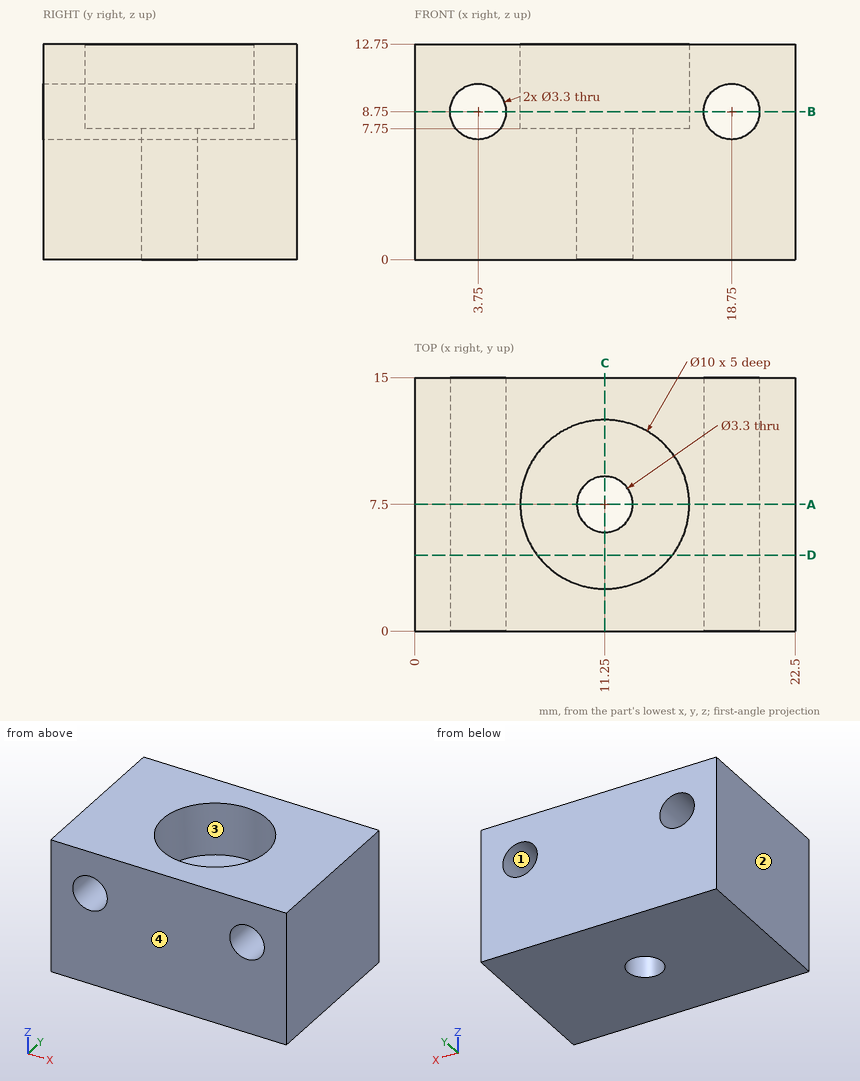
Geometry check sheet. Reference: drawing and pictorial views, mm from the part's lowest x, y, z. Coordinates: 2 decimals unless noted, no trailing zeros. Order: outer loops, then holes, each group sorted by start corner. A loop starts at its lowest first (then second) coordinate and runs counter-clockwise, first axis right, second up.
Item 1: Mould release check, pull along X, two halves, no side actions. Record for the marked faces 1, 2, 3 and 4: released by +X, released by -X, zero draft, split by the parting line, or undercut.
Item 2: Section check A-A (y = 7.5). Enter the section's corners in (x, z).
Item 3: Section check D-D (y = 4.5). Enter the section's corners in (x, z).
Item 4: Scan lines: line 1 along X through (y, z) = (10.75, 8.75); line 2 along Y through (x, z) = (11.25, 10); line 3 along X through (y, z) = (7, 8.75). Record each from-to range of solid material in increasing order.
Item 5: Section check B-B (z = 8.75). Enter the section's corners in (x, y), plus the area to 3 significant figures.
Item 6: Section check C-C (x = 11.25). Enter the section's corners in (y, z).
Check sheet entries:
1. face 1: undercut
1. face 2: released by -X
1. face 3: undercut
1. face 4: zero draft
2. outline: (0, 0) - (9.6, 0) - (9.6, 7.75) - (6.25, 7.75) - (6.25, 12.75) - (0, 12.75) - close; (12.9, 0) - (22.5, 0) - (22.5, 12.75) - (16.25, 12.75) - (16.25, 7.75) - (12.9, 7.75) - close; hole circle Ø3.3 at (3.75, 8.75); hole circle Ø3.3 at (18.75, 8.75)
3. outline: (0, 0) - (22.5, 0) - (22.5, 12.75) - (15.25, 12.75) - (15.25, 7.75) - (7.25, 7.75) - (7.25, 12.75) - (0, 12.75) - close; hole circle Ø3.3 at (3.75, 8.75); hole circle Ø3.3 at (18.75, 8.75)
4. line 1: x = 0 to 2.1, 5.4 to 7.45, 15.05 to 17.1, 20.4 to 22.5
4. line 2: y = 0 to 2.5, 12.5 to 15
4. line 3: x = 0 to 2.1, 5.4 to 6.28, 16.22 to 17.1, 20.4 to 22.5
5. outline: (0, 0) - (2.1, 0) - (2.1, 15) - (0, 15) - close; (5.4, 0) - (17.1, 0) - (17.1, 15) - (5.4, 15) - close; (20.4, 0) - (22.5, 0) - (22.5, 15) - (20.4, 15) - close; hole circle Ø10 at (11.25, 7.5)
5. area: 160 mm2
6. outline: (0, 0) - (5.85, 0) - (5.85, 7.75) - (2.5, 7.75) - (2.5, 12.75) - (0, 12.75) - close; (9.15, 0) - (15, 0) - (15, 12.75) - (12.5, 12.75) - (12.5, 7.75) - (9.15, 7.75) - close
